Read the model definition and answer for the solid it produces. Units are mm, in the model's axes. Face numbers are marked on the shaded views. A direction names the side the tool comes from. Give positions to 0.01 mm unless a question says otherwise; leave off trailing zeros. Order: outer loops, then holes, each group sorted by start corner. A loop starts at its lowest first (then second) coordinate and runs counter-clockwise, first axis right, second up.
```python
from build123d import *

# Parameters (mm, degrees)
F0_R           = 25.4
F1_DEPTH       = 6.35
F3_D           = 3.4
F3_CSINK_D     = 6.72
F3_CSINK_ANGLE = 90
F4_R           = 10.16
F5_DEPTH       = 9.525
F6_R           = 10.16
F6_R_2         = 10
F7_DEPTH       = 8
F8_R           = 6.35
F9_DEPTH       = 63.5


with BuildPart() as f1:
    # F0 (on Front) → F1 (new body)
    with BuildSketch(Plane.XZ):
        Circle(F0_R)
    extrude(amount=F1_DEPTH)

    # F3 (through all)
    with Locations(Plane.XZ.offset(6.35)):
        with Locations((-12.5, 12.059730643), (12.5, 12.059730643), (12.5, -12.059730643), (-12.5, -12.059730643)):
            CounterSinkHole(F3_D / 2, F3_CSINK_D / 2, counter_sink_angle=F3_CSINK_ANGLE)

    # F4 (on face) → F5 (join)
    with BuildSketch(Plane.XZ.offset(6.35)):
        Circle(F4_R)
    extrude(amount=F5_DEPTH)

    # F6 (on face) → F7 (cut)
    with BuildSketch(Plane.XZ.offset(15.875)):
        Circle(F6_R)
        Circle(F6_R_2, mode=Mode.SUBTRACT)
    extrude(amount=-F7_DEPTH, mode=Mode.SUBTRACT)

    # F8 (on face) → F9 (join)
    with BuildSketch(Plane.XZ.offset(15.875)):
        Circle(F8_R)
    extrude(amount=F9_DEPTH)


solid = f1.part
```
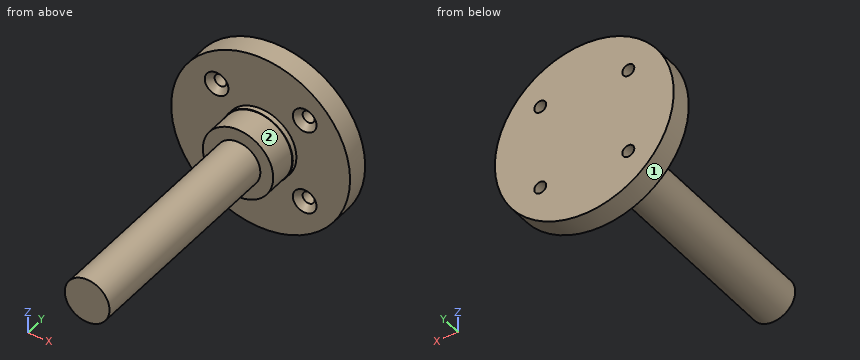
1) A tool of negligible diameter and unlimited length cuts with its end or side. For the marked faces 1 and 2, from which of +Z, -Z, +X, -X, +Y, -Y can it reach the whole face along a straight path? Write none if from no direction.
Final values:
face 1: +Y, -Y
face 2: -Y
2) Consider L1, parallel to Z at x = 12, y = -2; L2, parallel to Z at x = -12.5, y = -2; L3, parallel to Y at x = -21, z = 1. Determine where each line is inside the solid, lowest interval first.
Final values:
L1: z = -22.39 to -13.68, -10.43 to 10.43, 13.68 to 22.39
L2: z = -22.11 to -13.76, -10.36 to 10.36, 13.76 to 22.11
L3: y = -6.35 to 0
3) The part is cut by section B-B on z = 0. Determine the outline of the cut face in (x, y) (3 decimals), and give its area (3 significant figures).
Final values:
outline: (-25.4, -6.35) - (-10.16, -6.35) - (-10.16, -7.875) - (-10, -7.875) - (-10, -15.875) - (-6.35, -15.875) - (-6.35, -79.375) - (6.35, -79.375) - (6.35, -15.875) - (10, -15.875) - (10, -7.875) - (10.16, -7.875) - (10.16, -6.35) - (25.4, -6.35) - (25.4, 0) - (-25.4, 0) - close
area: 1,320 mm2
4) The part is cut by section C-C on x = 12.5. Determine the outline of the cut face in (y, z), and give its area (3 significant figures).
Final values:
outline: (-6.35, -22.11) - (0, -22.11) - (0, -13.76) - (-4.69, -13.76) - (-6.35, -15.42) - close; (-6.35, -8.7) - (-4.69, -10.36) - (0, -10.36) - (0, 10.36) - (-4.69, 10.36) - (-6.35, 8.7) - close; (-6.35, 15.42) - (-4.69, 13.76) - (0, 13.76) - (0, 22.11) - (-6.35, 22.11) - close
area: 232 mm2
5) Given pin 1 (5.5 mm diameter, centred on x = 12.5, z = 12.06, fed in from -Y); pin 2 (4 mm diameter, centred on x = -6, z = -6, fed in from -Y) (3 decimals); pin 3 (10 mm diameter, centred on x = -9.5, y = -36, fed in from +Z), each flat-ended and moving along its own axis, determine where each tip first touches the part or whether it passes through.
Final values:
pin 1: stops at y = -5.74
pin 2: stops at y = -15.875
pin 3: stops at z = 4.48
6) The part is cut by section D-D on y = -69.5. Determine the outline of the cut face in (x, z), and give its area (3 significant figures).
Final values:
outline: circle Ø12.7 at (0, 0)
area: 127 mm2
7) The part is cut by section A-A on x = 0. Determine the outline of the cut face in (y, z) (3 decimals), and give its area (3 significant figures).
Final values:
outline: (-79.375, -6.35) - (-15.875, -6.35) - (-15.875, -10) - (-7.875, -10) - (-7.875, -10.16) - (-6.35, -10.16) - (-6.35, -25.4) - (0, -25.4) - (0, 25.4) - (-6.35, 25.4) - (-6.35, 10.16) - (-7.875, 10.16) - (-7.875, 10) - (-15.875, 10) - (-15.875, 6.35) - (-79.375, 6.35) - close
area: 1,320 mm2
